Verification items for this drawing (mm, ordinates from the low corner). A direction names the side the tool comes from. Round coordinates to 2 decimals unless told otherwise and drop trailing zeros. Order: outer loops, then holes, each group sorted by start corner. A loop starts at its lowest first (then second) coordinate and runs counter-clockwise, first axis right, second up. Notation, with made-up numbers: M 52,15 L 83,15 A26 ccw 83,47 Z; hole C 61.5,55.5 d2. An arc over 180 degrees is marked long. Return JSON: item names as keys, results as strings. Group by question number.
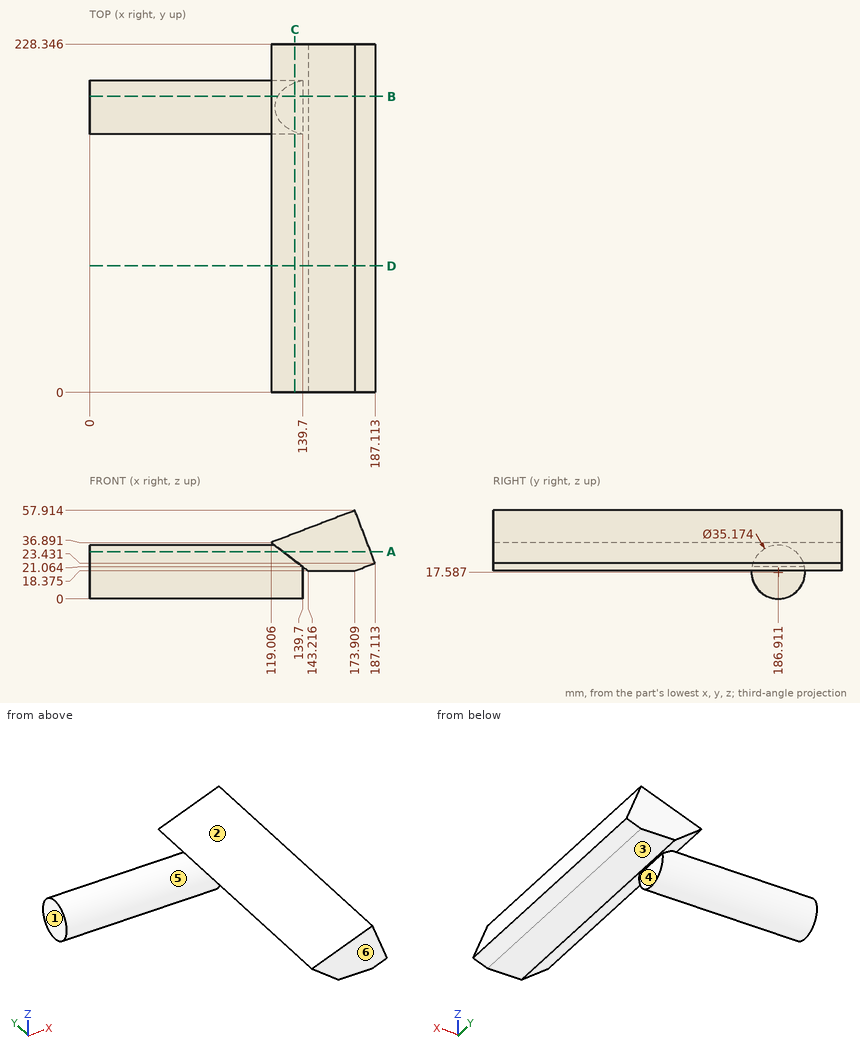
1. Cross-section at A-A (z = 31). Enter the section's corners in (x, y) (1 decimal), plus the area to 3 significant figures.
2. Draft check along Z on the marked faces 1, 2 and 3. Enter one of: +Z half, -Z half, draft (parallel to the pull), parting line (faces both ways), or undercut.
3. Cross-section at D-D (y = 83). Enter the section's corners in (x, z) (1 decimal).
4. Cross-section at C-C (x = 134.5). Enter the section's corners in (y, z), plus the area to 3 significant figures.
5. Access from +Z, -Z, +X, -X, +Y, -Y to the whole of each face (thin tool, end or side, straight path). Record for the marked faces 4, 5 and 6.
6. Cross-section at B-B (y = 194). Enter the section's corners in (x, z) (1 decimal).
7. Go/stop test with flat-tipped pins: pin 1 (10 mm diameter, centred on x = 120, y = 179.5, fed in from +Z); pin 2 (5 mm diameter, centred on x = 156, y = 111.5, fed in from -Z) (1 decimal); pin 3 (4 mm diameter, centred on x = 73.5, z = 32, fed in from -Y). Record where each tip stops, or that it passes through.
8. Thickness scan on line 1 along X through (y, z) = (180, 9.5); line 2 along Y through (x, z) = (55, 32) (1 decimal); line 3 along Y through (x, z) = (110, 5.5) (1 decimal). Record the ranges inside material, lowest first. Write a range as from..to.
Computed:
{
 "1": {"outline": "M 0,175.5 L 126.7,175.5 L 126.7,0 L 184.2,0 L 184.2,228.3 L 126.7,228.3 L 126.7,198.3 L 0,198.3 Z", "area": "16,000 mm²"},
 "2": {"face 1": "draft", "face 2": "+Z half", "face 3": "-Z half"},
 "3": {"outline": "M 119,36.9 L 143.2,18.4 L 173.9,18.4 L 187.1,23.4 L 173.9,57.9 Z"},
 "4": {"outline": "M 0,25.04 L 170.98,25.04 A17.59 ccw long 202.84,25.04 L 228.35,25.04 L 228.35,42.82 L 0,42.82 Z", "area": "4,800 mm²"},
 "5": {"face 4": "-Z, +Y, -Y", "face 5": "-X", "face 6": "+Z, -Z, +X, -X, -Y"},
 "6": {"outline": "M 0,1.5 L 139.7,1.5 L 139.7,21.1 L 143.2,18.4 L 173.9,18.4 L 187.1,23.4 L 173.9,57.9 L 119,36.9 L 123.2,33.7 L 0,33.7 Z"},
 "7": {"pin 1": "stops at z = 39.19", "pin 2": "stops at z = 18.4", "pin 3": "stops at y = 174.45"},
 "8": {"line 1": "x = 0..139.7", "line 2": "y = 176.8..197", "line 3": "y = 174.1..199.7"}
}
